Here's how the part is built. I have some questions about the finished solid (model axes, mm). A direction names the side the tool comes from. Give positions to 0.01 mm unless a question says otherwise; leave off trailing zeros. Write each loop counter-clockwise with the first axis right and the second up, starting at its lowest first coordinate (ties: lowest second). Pieces come first, ordered by that corner, then holes. Notation, with made-up numbers: (24, 18.25) -> (38, 18.25) arc R30 cw to (38, 53.25) -> close; hole circle Ø1 at (-7, -32.75). An arc over 180 degrees is marked (long way). Use one line per item in the form item = value.
```python
from build123d import *

# Parameters (mm, degrees)
F0_W     = 984.25
F0_H     = 622.3
F1_DEPTH = 177.8
F2_W     = 984.25
F2_H     = 622.3
F3_DEPTH = 19.05
F0_W_2   = 946.15
F0_H_2   = 19.05
F4_DEPTH = 177.8
F6_DEPTH = 984.25


with BuildPart() as f1:
    # F0 (on Front) → F1 (new body)
    with BuildSketch(Plane.XZ):
        Rectangle(F0_W, F0_H)
        Polygon((473.075, -292.1), (-473.075, -292.1), (-473.075, -9.525), (-473.075, 9.525), (-473.075, 292.1), (473.075, 292.1), (473.075, 9.525), (473.075, -9.525), align=None, mode=Mode.SUBTRACT)
    extrude(amount=-F1_DEPTH)

    # F2 (on face) → F3 (join)
    with BuildSketch(Plane(origin=(0, 177.8, 0), x_dir=(-1, 0, 0), z_dir=(0, 1, 0))):
        Rectangle(F2_W, F2_H)
    extrude(amount=F3_DEPTH)

    # F0 (on Front) → F4 (join)
    with BuildSketch(Plane.XZ):
        Rectangle(F0_W_2, F0_H_2)
    extrude(amount=-F4_DEPTH)

    # F5 (on face) → F6 (join)
    with BuildSketch(Plane.YZ.offset(492.125)):
        Polygon((215.9, 285.75), (196.85, 285.75), (196.85, 250.825), (212.725, 234.95), (215.9, 234.95), align=None)
        Polygon((215.9, -171.45), (196.85, -171.45), (196.85, -206.375), (212.725, -222.25), (215.9, -222.25), align=None)
    extrude(amount=-F6_DEPTH)


solid = f1.part
```
Q1. Which directions (+Z, -Z, +X, -X, +Y, -Y) give clear straight access to the entire face, cutting with the end or side of a thin tool? Please do faces 1 (the face through (7, 207, -171.45)), 2 (the face through (7, 177.8, -149)), 3 (the face through (7, 196.85, 299)), 4 (the face through (-148, 0, 1)).
Result set:
face_1 = +X, -X, +Y
face_2 = -Y
face_3 = +Z, +X, -X, +Y
face_4 = +Z, -Z, +X, -X, -Y
Q2. I want a section at C-C, the plane x = 385.5. Write out the boundary of the cut face in (y, z) (3 decimals).
Result set:
outline = (0, -311.15) -> (196.85, -311.15) -> (196.85, -206.375) -> (212.725, -222.25) -> (215.9, -222.25) -> (215.9, -171.45) -> (196.85, -171.45) -> (196.85, 250.825) -> (212.725, 234.95) -> (215.9, 234.95) -> (215.9, 285.75) -> (196.85, 285.75) -> (196.85, 311.15) -> (0, 311.15) -> (0, 292.1) -> (177.8, 292.1) -> (177.8, 9.525) -> (0, 9.525) -> (0, -9.525) -> (177.8, -9.525) -> (177.8, -292.1) -> (0, -292.1) -> close
Q3. If we mould it in two halves opening along Z, with no side actions, what happens to faces 5 (the face through (7, 97, 311.15)), 6 (the face through (-7, 88, 292.1)), 7 (the face through (7, 196.85, -258)), 8 (the face through (-473.075, 88, 149))? For each: +Z half, -Z half, draft (parallel to the pull), parting line (faces both ways), or undercut.
Result set:
face_5 = +Z half
face_6 = undercut
face_7 = draft
face_8 = undercut
Q4. I want a section at A-A, the plane y = 151.5. Write out the boundary of the cut face in (x, z) (3 decimals), and give its area (3 significant figures).
Result set:
outline = (-492.125, -311.15) -> (492.125, -311.15) -> (492.125, 311.15) -> (-492.125, 311.15) -> close; hole (-473.075, -292.1) -> (473.075, -292.1) -> (473.075, -9.525) -> (-473.075, -9.525) -> close; hole (-473.075, 9.525) -> (473.075, 9.525) -> (473.075, 292.1) -> (-473.075, 292.1) -> close
area = 77,800 mm2
Q5. If I drill on line 1 along Z through (x, y) = (138, 154.5) (3 decimals); line 2 along X through (y, z) = (155, 259.5) (3 decimals); line 3 along Y through (x, z) = (-121.5, 167), over which ranges is the centre line in solid material (lowest first)? Write a range as from..to.
Result set:
line_1 = -311.15..-292.1, -9.525..9.525, 292.1..311.15
line_2 = -492.125..-473.075, 473.075..492.125
line_3 = 177.8..196.85
Q6. Will these pins go through, and if not, where does the flat tip stop? pin 1 Ø15 at (x, y) = (-231.5, 208.5) entering from +Z; pin 2 Ø3 at (x, z) = (312, -188.5) entering from -Y; pin 3 Ø2.5 at (x, y) = (149, 214) entering from -Z.
Result set:
pin_1 = 285.75
pin_2 = 177.8
pin_3 = -222.25
Q7. I want a section at B-B, the plane z = -73.5. Write out the boundary of the cut face in (x, y) (3 decimals).
Result set:
outline = (-492.125, 0) -> (-473.075, 0) -> (-473.075, 177.8) -> (473.075, 177.8) -> (473.075, 0) -> (492.125, 0) -> (492.125, 196.85) -> (-492.125, 196.85) -> close
